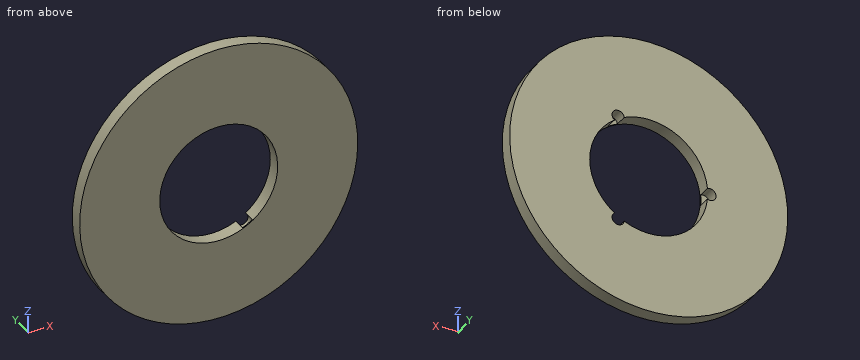
from build123d import *

# Parameters (mm, degrees)
SKETCH1_R           = 82.5
BOSS_EXTRUDE1_DEPTH = 8
SKETCH2_R           = 35
CUT_EXTRUDE1_DEPTH  = 117.946568996
SKETCH3_R           = 3.621742951
CUT_EXTRUDE2_DEPTH  = 7.301639
CIRPATTERN1_START   = 0.698361094
CIRPATTERN1_DEPTH   = 7.301638906


# Read off the part's stored shape, not the designer's step: CirPattern1
with BuildPart() as part:
    # Sketch1 → Boss-Extrude1 (new body)
    with BuildSketch(Plane(origin=(0, 0, 0), x_dir=(1, 0, 0), z_dir=(0, 1, 0))):
        with Locations(Location((0, 0, 0), (0, 0, 270))):
            Circle(SKETCH1_R)
    extrude(amount=BOSS_EXTRUDE1_DEPTH)

    # Sketch2 → Cut-Extrude1 (cut, through all)
    with BuildSketch(Plane(origin=(0, 0, 0), x_dir=(1, 0, 0), z_dir=(0, 1, 0))):
        with Locations(Location((0, 0, 0), (0, 0, 270))):
            Circle(SKETCH2_R)
    extrude(amount=CUT_EXTRUDE1_DEPTH, mode=Mode.SUBTRACT)

    # Sketch3 → Cut-Extrude2 (cut)
    with BuildSketch(Plane(origin=(0, 8, 0), x_dir=(1, 0, 0), z_dir=(0, 1, 0))):
        with Locations((-36.31964846, 0)):
            Circle(SKETCH3_R)
    extrude(amount=-CUT_EXTRUDE2_DEPTH, mode=Mode.SUBTRACT)

    # CirPattern1 outline → CirPattern1 (cut)
    with BuildSketch(Plane(origin=(0, 0, 0), x_dir=(1, 0, 0), z_dir=(0, 1, 0)).offset(CIRPATTERN1_START)):
        with BuildLine():
            ThreePointArc((14.557562001, 31.828876647), (17.5, 30.310889133), (20.285834749, 28.521656834))
            ThreePointArc((20.285834749, 28.521656834), (19.970695704, 34.590259624), (14.557562001, 31.828876647))
        make_face()
        with BuildLine():
            ThreePointArc((20.285834749, -28.521656834), (17.5, -30.310889133), (14.557562001, -31.828876647))
            ThreePointArc((14.557562001, -31.828876647), (19.970695704, -34.590259624), (20.285834749, -28.521656834))
        make_face()
    extrude(amount=CIRPATTERN1_DEPTH, mode=Mode.SUBTRACT)


solid = part.part
Can you work these out from the model? Positions are in its coordinate system, mm. Round coordinates to 2 decimals unless told otherwise and drop trailing zeros. Write each loop counter-clockwise with the first axis right and the second up, starting at its lowest first coordinate (ties: lowest second). Pieces come first, ordered by that corner, then holes. Notation, with made-up numbers: M 10.5,-12 L 55.5,-12 A27 ccw 55.5,14 Z; hole C 45,8 d6. An arc over 180 degrees is marked long. Use a Markdown table: item, result.
Item 1: I want a section at B-B (x = 0). List the corners of the cut face in (y, z) for me.
Found:
| item | result |
|---|---|
| outline | M 0,-82.5 L 8,-82.5 L 8,-35 L 0,-35 Z; M 0,35 L 8,35 L 8,82.5 L 0,82.5 Z |
Item 2: I want a section at A-A (z = 0). List the corners of the cut face in (x, y) for me, and give its area (3 significant figures).
Found:
| item | result |
|---|---|
| outline | M -82.5,0 L -35,0 L -35,0.7 L -39.94,0.7 L -39.94,8 L -82.5,8 Z; M 35,0 L 82.5,0 L 82.5,8 L 35,8 Z |
| area | 724 mm2 |
Item 3: I want a section at D-D (x = -26). List the corners of the cut face in (y, z) for me.
Found:
| item | result |
|---|---|
| outline | M 0,-78.3 L 8,-78.3 L 8,-23.43 L 0,-23.43 Z; M 0,23.43 L 8,23.43 L 8,78.3 L 0,78.3 Z |
Item 4: I want a section at C-C (y = 6.25). List the corners of the cut face in (x, z) for me, and give its area (3 significant figures).
Found:
| item | result |
|---|---|
| outline | C 0,0 d165; hole M -34.84,-3.31 A35 ccw 14.56,-31.83 A3.62 ccw long 20.29,-28.52 A35 ccw 20.29,28.52 A3.62 ccw long 14.56,31.83 A35 ccw -34.84,3.31 A3.62 ccw long Z |
| area | 17,400 mm2 |
Item 5: For pin 1 Ø6.5 at (x, z) = (-36.32, 0) entering from +Y; pin 2 Ø2 at (y, z) = (3.5, -47) entering from +X; pin 3 Ø4 at (x, y) = (-48, 5.5) entering from -Z, each with a flat end and sliding along its axis, tell me the tip position at first contact or that it passes through.
Found:
| item | result |
|---|---|
| pin 1 | stops at y = 0.7 |
| pin 2 | stops at x = 68.49 |
| pin 3 | stops at z = -68.49 |
Item 6: If I drill on line 1 along X through (y, z) = (6, 0); line 2 along X through (y, z) = (5.5, 22); line 3 along Z through (x, y) = (22.5, 2), over which ranges is the centre line in solid material (lowest first)? Write a range as [from, to].
Found:
| item | result |
|---|---|
| line 1 | x = [-82.5, -39.94], [35, 82.5] |
| line 2 | x = [-79.51, -27.22], [27.22, 79.51] |
| line 3 | z = [-79.37, -26.81], [26.81, 79.37] |
